Answer from the drawing. Dimensions are ordinates in mm from the lowest x, y and z of the part. A direction names the side the tool comes from. Give positions to 0.01 mm unless a question says otherwise; leave off trailing zeros. Loops run counter-clockwise (first coordinate to the right, second up) from the corner with the lowest first, then second, coordinate; pieces in that order, holes last.
Item 1: Section B-B, the plane z = 8.89 is taken. Give the vertices of the cut face in (x, y), and give its area (3 significant figures).
Item 2: Section D-D, the plane y = 4.5 is taken. Give the vertices of the cut face in (x, z), and give its area (3 significant figures).
Item 3: A tool of negligible diameter and unlimited length cuts with its end or side. For the marked faces 5 and 6, from which of +Z, -Z, +X, -X, +Y, -Y can it reach the whole face along a straight path? Write none if from no direction.
Item 4: The mould has two halves that part along Y. Classify the marked faces 1, 2, 3 and 4: pulls with the +Y half, pulls with the -Y half, needs draft (parallel to the pull), parting line crosses it, or undercut.
Item 5: Consider line 1 along Y through (x, z) = (7.62, 1.9); line 2 along Z through (x, y) = (7.62, 2.85); line 3 along Z through (x, y) = (7.62, 1.15). Determine where each line is inside the solid, lowest interval first.
Item 6: Section A-A, the plane y = 8.89 is taken. Give the vertices of the cut face in (x, z).
Item 7: Each of these flat-tipped pins is pushed along its axis until it touches: pin 1 Ø3 at (x, z) = (7.5, 7.5) entering from +Y; pin 2 Ø6 at (x, z) = (5, 11.5) entering from +Y; pin 3 Ø7.5 at (x, y) = (11, 11) entering from +Z. Where does it stop, or does it pass through?
Item 8: Section C-C, the plane x = 7.62 is taken. Give the vertices of the cut face in (y, z), and give its area (3 significant figures).
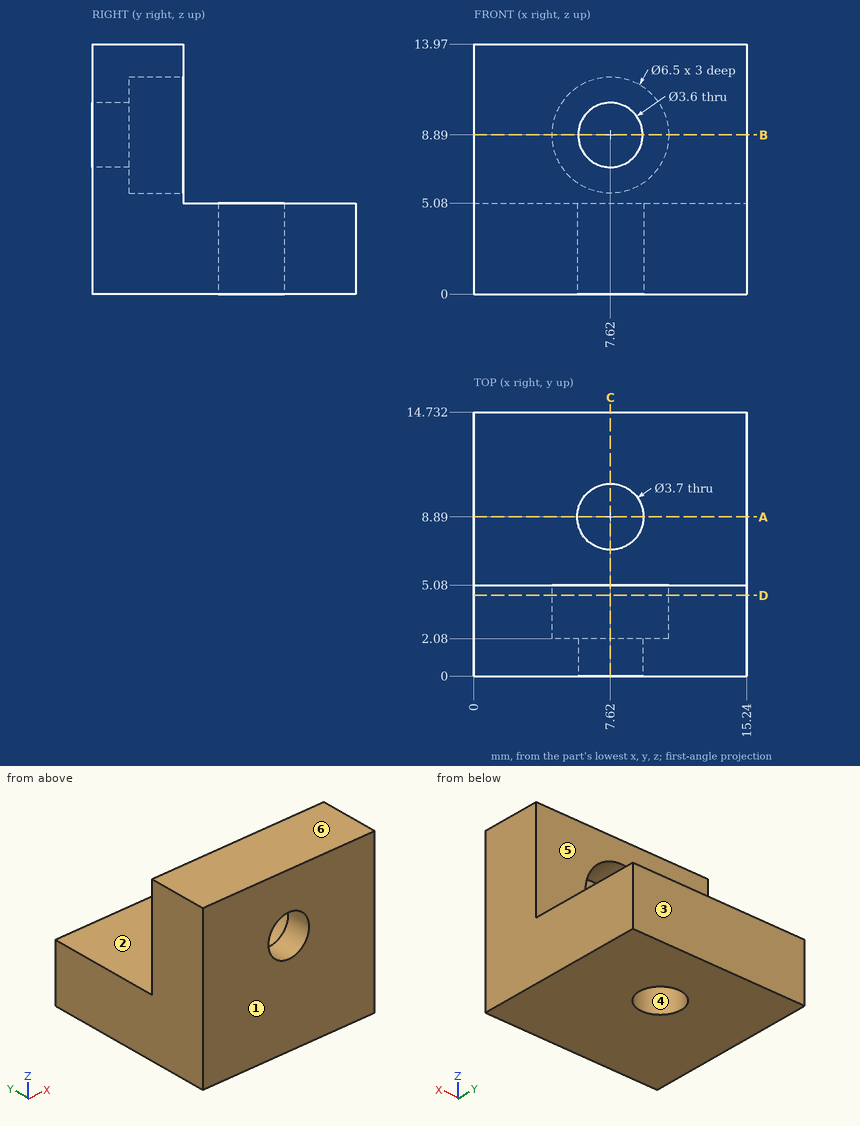
Worked answers:
1. outline: (0, 0) - (5.82, 0) - (5.82, 2.08) - (4.37, 2.08) - (4.37, 5.08) - (0, 5.08) - close; (9.42, 0) - (15.24, 0) - (15.24, 5.08) - (10.87, 5.08) - (10.87, 2.08) - (9.42, 2.08) - close
1. area: 50.4 mm2
2. outline: (0, 0) - (15.24, 0) - (15.24, 13.97) - (0, 13.97) - close; hole circle Ø6.5 at (7.62, 8.89)
2. area: 180 mm2
3. face 5: +Z, +X, -X, +Y
3. face 6: +Z, +X, -X, +Y, -Y
4. face 1: pulls with the -Y half
4. face 2: needs draft
4. face 3: pulls with the +Y half
4. face 4: undercut
5. line 1: y = 0 to 7.04, 10.74 to 14.73
5. line 2: z = 0 to 5.64, 12.14 to 13.97
5. line 3: z = 0 to 7.09, 10.69 to 13.97
6. outline: (0, 0) - (5.77, 0) - (5.77, 5.08) - (0, 5.08) - close; (9.47, 0) - (15.24, 0) - (15.24, 5.08) - (9.47, 5.08) - close
7. pin 1: stops at y = 2.08
7. pin 2: stops at y = 5.08
7. pin 3: stops at z = 5.08
8. outline: (0, 0) - (7.04, 0) - (7.04, 5.08) - (5.08, 5.08) - (5.08, 5.64) - (2.08, 5.64) - (2.08, 7.09) - (0, 7.09) - close; (0, 10.69) - (2.08, 10.69) - (2.08, 12.14) - (5.08, 12.14) - (5.08, 13.97) - (0, 13.97) - close; (10.74, 0) - (14.73, 0) - (14.73, 5.08) - (10.74, 5.08) - close
8. area: 74.2 mm2
